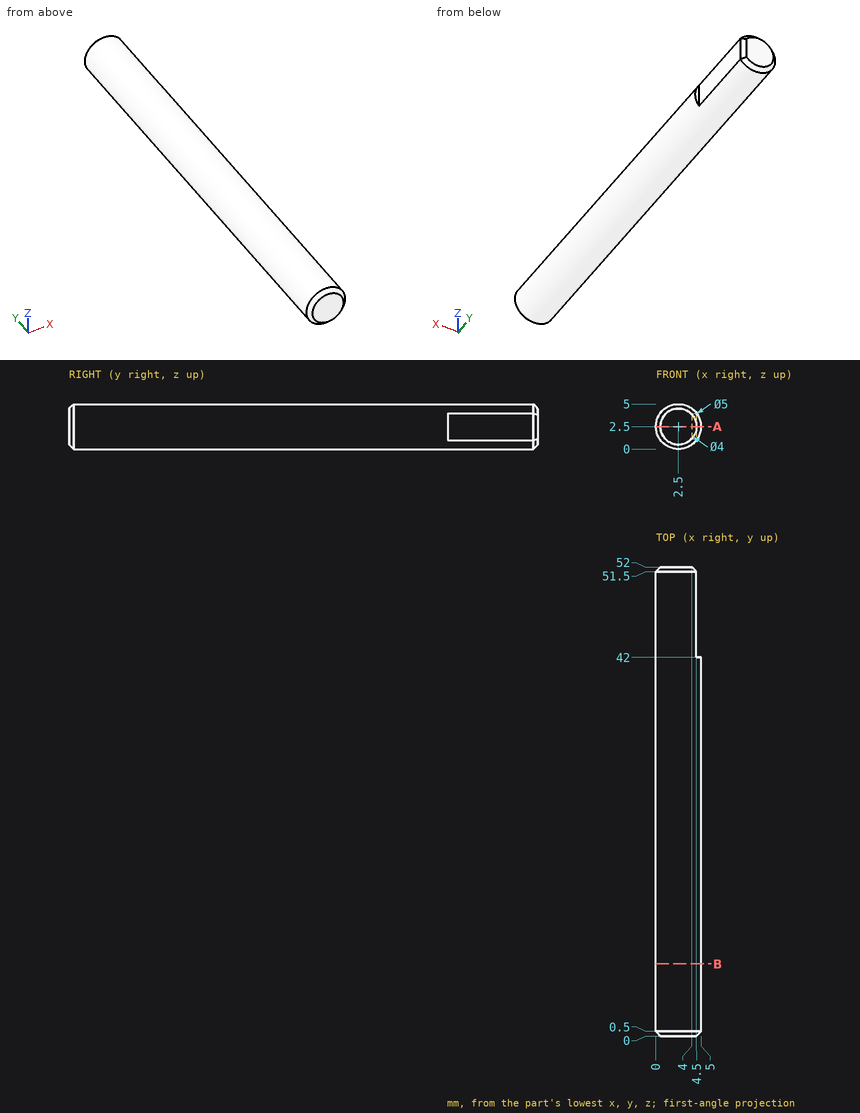
Input: dimensioned drawing with shaded views. Units: mm. Origin: part minimum x, y, z. Coordinates: 2 decimals unless noted, no trailing zeros. Loops run counter-clockwise (first coordinate to the right, second up) from the corner with the lowest first, then second, coordinate; pieces in that order, holes last. Notation, with made-up numbers: (27.25, 43.25) - (55.25, 43.25) arc R6 cw to (55.25, 50.25) - close; hole circle Ø7 at (-14, 71). An arc over 180 degrees is marked (long way). One line per question, with ' | ' between items. Start each with the question number.
(1) Cut plane B-B on y = 8. Output: boundary loops of the cut face in (x, z).
(2) Ray query, L1, parallel to X at y = 28.5, z = 2.35; L2, parallel to X at y = 35, z = 3.35; L3, parallel to Y at x = 0.75, z = 0.95. Return the intervals inside material, ascending. Write a range as from..to.
(3) Cut plane A-A on z = 2.5. Output: boundary loops of the cut face in (x, y), and give its area (4 significant figures).
Here are the results:
1) outline: circle Ø5 at (2.5, 2.5)
2) L1: 0..5 | L2: 0.15..4.85 | L3: 0.34..51.66
3) outline: (0, 0.5) - (0.5, 0) - (4.5, 0) - (5, 0.5) - (5, 42) - (4.5, 42) - (4.5, 51.5) - (4, 52) - (0.5, 52) - (0, 51.5) - close | area: 254.5 mm²
